Source: three-view drawing plus pictorial views. Frame: mm from the lowest corner of the part. A direction names the side the tool comes from. Give positions to 0.01 mm unless a question says otherwise; leave off trailing zeros. Loops run counter-clockwise (first coordinate to the right, second up) from the corner with the lowest first, then second, coordinate; pieces in that order, holes last. Notation, with made-up numbers: (30, 23) -> (69, 23) arc R30 ccw to (69, 47) -> close; hole circle Ø2 at (36.5, -18). An arc over 180 degrees is marked (long way). Answer as a JSON object with one key per item and string values. Group by question number.
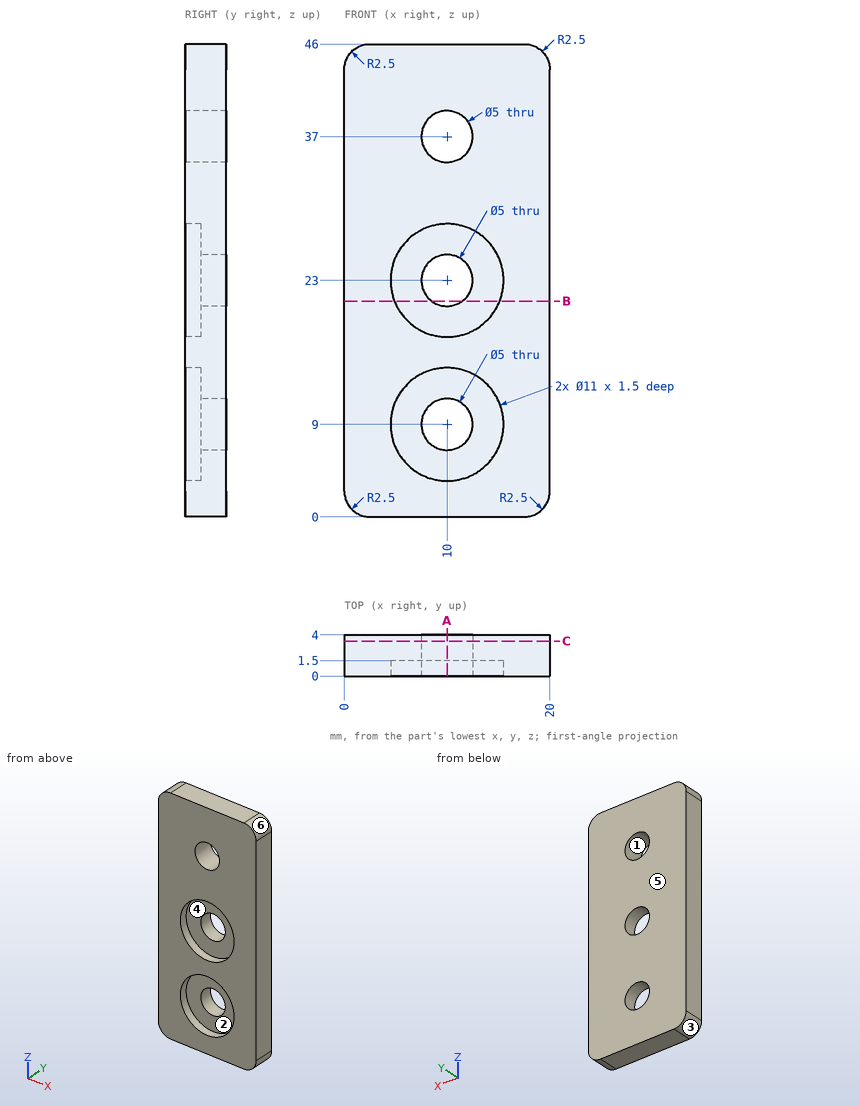
(1) Section query B-B on z = 21. Return the cut outline in (x, y), plus the area to 3 significant figures.
(2) First-contact query: pin 1 (4 mm diameter, centred on x = 10, z = 9, fed in from +Y); pin 2 (6.5 mm diameter, centred on x = 10, z = 9, fed in from -Y). Flat tips, straight axial feed; report the tip coordinate or a pass-through.
(3) Section query C-C on y = 3.4. Return the cut outline in (x, z).
(4) Access query for the marked faces 1 and 2. Directions: +Z, -Z, +X, -X, +Y, -Y. A direction counts if a zero-diameter tool reaches every point of the face in a straight line with its end or side. Return the directions, or none.
(5) Mould query, pull axis X, two halves, no side actions, for the marked faces 3, 4, 5 and 6. Classes: pulls with the +X half, pulls with the -X half, needs draft (parallel to the pull), parting line crosses it, or undercut.
(6) Material intervals for line 1 (Z direction, x = 10, y = 2); line 2 (Z direction, x = 10, y = 1.05); line 3 (X direction, y = 2.35, z = 23), sorted ascending. Write a range as from..to.
(7) Section query A-A on x = 10. Return the cut outline in (y, z).
Result:
{
 "1": {"outline": "(0, 0) -> (4.88, 0) -> (4.88, 1.5) -> (8.5, 1.5) -> (8.5, 4) -> (0, 4) -> close; (11.5, 1.5) -> (15.12, 1.5) -> (15.12, 0) -> (20, 0) -> (20, 4) -> (11.5, 4) -> close", "area": "57.1 mm²"},
 "2": {"pin 1": "through", "pin 2": "y = 1.5"},
 "3": {"outline": "(0, 2.5) arc R2.5 ccw to (2.5, 0) -> (17.5, 0) arc R2.5 ccw to (20, 2.5) -> (20, 43.5) arc R2.5 ccw to (17.5, 46) -> (2.5, 46) arc R2.5 ccw to (0, 43.5) -> close; hole circle Ø5 at (10, 9); hole circle Ø5 at (10, 23); hole circle Ø5 at (10, 37)"},
 "4": {"face 1": "+Y, -Y", "face 2": "-Y"},
 "5": {"face 3": "pulls with the -X half", "face 4": "undercut", "face 5": "needs draft", "face 6": "pulls with the +X half"},
 "6": {"line 1": "0..6.5, 11.5..20.5, 25.5..34.5, 39.5..46", "line 2": "0..3.5, 14.5..17.5, 28.5..34.5, 39.5..46", "line 3": "0..7.5, 12.5..20"},
 "7": {"outline": "(0, 0) -> (4, 0) -> (4, 6.5) -> (1.5, 6.5) -> (1.5, 3.5) -> (0, 3.5) -> close; (0, 14.5) -> (1.5, 14.5) -> (1.5, 11.5) -> (4, 11.5) -> (4, 20.5) -> (1.5, 20.5) -> (1.5, 17.5) -> (0, 17.5) -> close; (0, 28.5) -> (1.5, 28.5) -> (1.5, 25.5) -> (4, 25.5) -> (4, 34.5) -> (0, 34.5) -> close; (0, 39.5) -> (4, 39.5) -> (4, 46) -> (0, 46) -> close"}
}
